from build123d import *

# Parameters (mm, degrees)
F2_R     = 4.5
F3_DEPTH = 12
F5_DEPTH = 10


with BuildPart() as f1:
    # F0 (on Top) → F1 (revolve)
    with BuildSketch(Plane.XY):
        with BuildLine():
            Line((-6.456904, -3), (-6.75, 0))
            Line((-6.75, 0), (-8.75, 0))
            Line((-8.75, 0), (-7.816054, -8.225632))
            ThreePointArc((-7.816054, -8.225632), (-7.160877, -9.491855), (-5.828823, -10))
            Line((-5.828823, -10), (0, -10))
            Line((0, -10), (0, -3))
            Line((0, -3), (-6.456904, -3))
        make_face()
    revolve(axis=Axis((0, -5, 0), (0, -1, 0)))

    # F2 (on face) → F3 (join)
    with BuildSketch(Plane(origin=(0, -3, 0), x_dir=(-1, 0, 0), z_dir=(0, 1, 0))):
        Circle(F2_R)
    extrude(amount=F3_DEPTH)

    # F4 (on face) → F5 (cut)
    with BuildSketch(Plane(origin=(0, 9, 0), x_dir=(-1, 0, 0), z_dir=(0, 1, 0))):
        with BuildLine():
            Line((-2.50998, -1.55), (2.50998, -1.55))
            ThreePointArc((2.50998, -1.55), (0, 2.95), (-2.50998, -1.55))
        make_face()
    extrude(amount=-F5_DEPTH, mode=Mode.SUBTRACT)


solid = f1.part
Geometry check sheet. Reference: the model listing, model coordinates, mm. A direction names the side the tool comes from. Round coordinates to 2 decimals unless told otherwise and drop trailing zeros. Order: outer loops, then holes, each group sorted by start corner. A loop starts at its lowest first (then second) coordinate and runs counter-clockwise, first axis right, second up. Notation, with made-up numbers: M 52.25,69.25 L 64.25,69.25 A22 cw 64.25,100.25 Z; hole C 74.25,-24.75 d7. An arc over 180 degrees is marked long. Write each question's results on one line, items separated by ' | '. Start each with the question number.
1. Cross-section at C-C on y = -0.75. Record the boundary of the cut face in (x, z).
2. Set-up check for faces 4 (the face through (-1.525, -3, -4.395)), 5 (the face through (0, 9, -2)): record each of +Z, -Z, +X, -X, +Y, -Y from which the full face is reachable in a straight line by a thin tool's end or side.
3. Cross-section at A-A on x = 0. Record the boundary of the cut face in (y, z).
4. Draft check along X on faces 1 (the face through (0, -10, 0)), 2 (the face through (1.064, -5.084, -8.103)), 3 (the face through (0, 4, -1.55)). Enter one of: pulls with the +X half, pulls with the -X half, needs draft (parallel to the pull), parting line crosses it, or undercut.
5. Cross-section at B-B on z = 0. Record the boundary of the cut face in (x, y), plus the area to 3 significant figures.
6. Go/stop test with flat-tipped pins: P1, Ø5.5, axis at x = 0.5, y = 4, coming from the +Z side; P2, Ø3, axis at x = -6, z = 6, coming from the -Y side; P3, Ø3, axis at y = -7, z = 0, coming from the +X side. Record where each tip stops, or that it passes through.
7. Cross-section at D-D on y = 2.5. Record the boundary of the cut face in (x, z), plus the area to 3 significant figures.
8. Material ranges on L1, parallel to Z at x = 3, y = -2.5; L2, parallel to X at y = -0.25, z = 1.5; L3, parallel to Y at x = -1.5, z = 1.25, recorded low to high. Write a range as from..to.
Resolved:
1) outline: C 0,0 d17.33; C 0,0 d9; hole C 0,0 d13.35; hole M -2.51,-1.55 L 2.51,-1.55 A2.95 ccw long Z
2) face 4: +Y | face 5: +Z, -Z, +X, -X, +Y
3) outline: M -10,-5.83 A2 ccw -8.23,-7.82 L 0,-8.75 L 0,-6.75 L -3,-6.46 L -3,-4.5 L 9,-4.5 L 9,-1.55 L -1,-1.55 L -1,2.95 L 9,2.95 L 9,4.5 L -3,4.5 L -3,6.46 L 0,6.75 L 0,8.75 L -8.23,7.82 A2 ccw -10,5.83 Z
4) face 1: needs draft | face 2: parting line crosses it | face 3: undercut
5) outline: M -8.75,0 L -7.82,-8.23 A2 ccw -5.83,-10 L 5.83,-10 A2 ccw 7.82,-8.23 L 8.75,0 L 6.75,0 L 6.46,-3 L 4.5,-3 L 4.5,9 L 2.95,9 L 2.95,-1 L -2.95,-1 L -2.95,9 L -4.5,9 L -4.5,-3 L -6.46,-3 L -6.75,0 Z | area: 172 mm2
6) P1: z = 4.5 | P2: y = -9.63 | P3: x = 8.13
7) outline: C 0,0 d9; hole M -2.51,-1.55 L 2.51,-1.55 A2.95 ccw long Z | area: 41.2 mm2
8) L1: -7.92..-5.77, -3.35..3.35, 5.77..7.92 | L2: -8.59..-6.56, -4.24..-2.54, 2.54..4.24, 6.56..8.59 | L3: -10..-1
